Can you work these out from the model? Positions are in its coordinate system, mm. Face numbers are marked on the shaded views. A direction names the side the tool comes from. Round coordinates to 2 decimals unless told otherwise and drop trailing zeros. Loops run counter-clockwise (first coordinate to the right, second up) from the corner with the lowest first, then second, coordinate; pieces in that order, holes last. Notation, with made-up numbers: (-39.75, 54) -> (5.25, 54) arc R26 cw to (5.25, 77) -> close; hole circle Ø11 at (78, -27.5). An arc over 180 degrees is marked (long way). Write item = value, one per line.
from build123d import *

# Parameters (mm, degrees)
SKETCH1_R           = 1.5
BOSS_EXTRUDE1_DEPTH = 2
BOSS_EXTRUDE2_DEPTH = 5


with BuildPart() as part:
    # Sketch1 → Boss-Extrude1 (new body)
    with BuildSketch(Plane(origin=(0, 0, 0), x_dir=(1, 0, 0), z_dir=(0, 1, 0))):
        with BuildLine():
            Line((2.25, -2.937260629), (14.03813079, -2.195659328))
            ThreePointArc((14.03813079, -2.195659328), (16.1, 0), (14.03813079, 2.195659328))
            Line((14.03813079, 2.195659328), (2.25, 2.937260629))
            ThreePointArc((2.25, 2.937260629), (-3.7, 0), (2.25, -2.937260629))
        make_face()
        with Locations(Location((0, 0, 0), (0, 0, 270))):
            Circle(SKETCH1_R, mode=Mode.SUBTRACT)
    extrude(amount=BOSS_EXTRUDE1_DEPTH)

    # Sketch1_3 → Boss-Extrude2 (add)
    with BuildSketch(Plane(origin=(0, 0, 0), x_dir=(1, 0, 0), z_dir=(0, 1, 0))):
        with BuildLine():
            Line((0.669064748, -6.163793666), (14.407194245, -4.672553263))
            ThreePointArc((14.407194245, -4.672553263), (18.6, 0), (14.407194245, 4.672553263))
            Line((14.407194245, 4.672553263), (0.669064748, 6.163793666))
            ThreePointArc((0.669064748, 6.163793666), (-6.2, 0), (0.669064748, -6.163793666))
        make_face()
        with BuildLine():
            ThreePointArc((14.03813079, -2.195659328), (16.1, 0), (14.03813079, 2.195659328))
            Line((14.03813079, 2.195659328), (2.25, 2.937260629))
            ThreePointArc((2.25, 2.937260629), (-3.7, 0), (2.25, -2.937260629))
            Line((2.25, -2.937260629), (14.03813079, -2.195659328))
        make_face(mode=Mode.SUBTRACT)
    extrude(amount=BOSS_EXTRUDE2_DEPTH)


solid = part.part
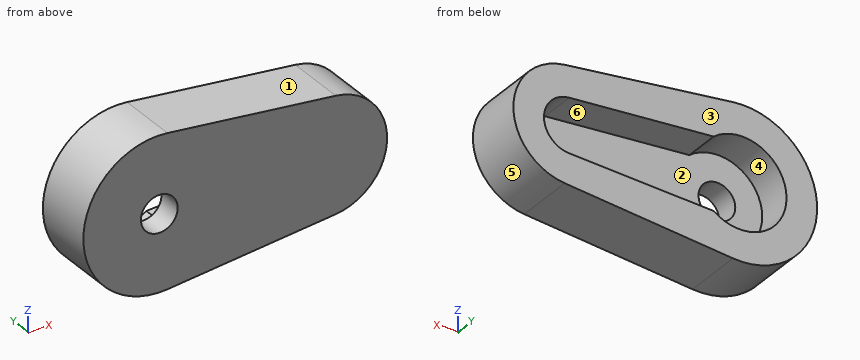
1. Suppose I cut it at A-A, the plane z = 0. List the corners of the cut face in (x, y) for me.
Entries:
outline = (-6.2, 0) -> (-1.5, 0) -> (-1.5, 2) -> (-3.7, 2) -> (-3.7, 5) -> (-6.2, 5) -> close; (1.5, 0) -> (18.6, 0) -> (18.6, 5) -> (16.1, 5) -> (16.1, 2) -> (1.5, 2) -> close
2. I'm going to push a flat-ended pin straight in: pin 1 (1 mm diameter, centred on y = 1.5, z = -3.5, fed in from +X). Where does the tip first touch, or does it pass through?
Entries:
pin_1 = 17.52
3. I need wall thicknesses on line 1 (Z direction, x = 0, y = 4.45); line 2 (Y direction, x = 1.5, z = -3); line 3 (Z direction, x = -2, y = 2.1). Which ranges of each line are inside material? Lowest first, please. Write a range as [from, to].
Entries:
line_1 = [-6.2, -3.7], [3.7, 6.2]
line_2 = [0, 2]
line_3 = [-5.87, -3.11], [3.11, 5.87]
4. For the marked faces 1 and 2, which set-ups out of +Z, -Z, +X, -X, +Y, -Y let a thin tool reach every point of the face, with its end or its side?
Entries:
face_1 = +Z, +X, +Y, -Y
face_2 = +Y
5. Suppose I cut it at B-B, the plane x = 0. List the corners of the cut face in (y, z) for me, and give its area (3 significant figures).
Entries:
outline = (0, -6.2) -> (5, -6.2) -> (5, -3.7) -> (2, -3.7) -> (2, -1.5) -> (0, -1.5) -> close; (0, 1.5) -> (2, 1.5) -> (2, 3.7) -> (5, 3.7) -> (5, 6.2) -> (0, 6.2) -> close
area = 33.8 mm²
6. We'd pull the mould along Z, two halves only. Please class the marked faces 3, 4, 5 and 6: released by +Z, released by -Z, zero draft, split by the parting line, or undercut.
Entries:
face_3 = zero draft
face_4 = undercut
face_5 = split by the parting line
face_6 = undercut
7. Suppose I cut it at C-C, the plane x = 2.5. List the corners of the cut face in (y, z) for me.
Entries:
outline = (0, -5.97) -> (5, -5.97) -> (5, -2.92) -> (2, -2.92) -> (2, 2.92) -> (5, 2.92) -> (5, 5.97) -> (0, 5.97) -> close
8. Suppose I cut it at D-D, the plane x = 5.5. List the corners of the cut face in (y, z) for me.
Entries:
outline = (0, -5.64) -> (5, -5.64) -> (5, -2.73) -> (2, -2.73) -> (2, 2.73) -> (5, 2.73) -> (5, 5.64) -> (0, 5.64) -> close
